Drawing for the job (mm, zero at the part's lowest x, y, z). A direction names the side the tool comes from. Coordinates: 2 decimals unless noted, no trailing zeros. Write each loop counter-clockwise with the first axis right and the second up, starting at its lowest first coordinate (ties: lowest second). Pieces come first, ordered by that corner, then holes. Notation, with made-up numbers: M 43,29.5 L 68,29.5 A27 cw 68,66.5 Z; hole C 81.25,-36 d4. An arc over 180 degrees is marked long. Use a Markdown table: item, result. Add a question column.
Q1. Tool access for the marked faces 5 and 6: list every direction of +Z, -Z, +X, -X, +Y, -Y with a clear straight run to the whole face (end or side of a thin tool).
Q2. Wall check: L1, parallel to X at y = 4, z = 19.05; L2, parallel to Z at x = 38.1, y = 3; L3, parallel to Z at x = 27, y = 13.5. Give the ranges that are in metal, low to high. Write a range as from..to.
Q3. Slice it at B-B on x = 38.1. Write the cut outline in (y, z).
Q4. Mould opens along Z. For the marked faces 1, 2, 3 and 4 say: released by +Z, released by -Z, zero draft, split by the parting line, or undercut.
Q5. Slice it at C-C on y = 17. Write the cut outline in (x, z).
Q6. Slice it at A-A on z = 19.05. Write the cut outline in (x, y), then the cut area to 3 significant figures.
Q7. Pin check, flat tips, straight feed: pin 1 Ø3 at (y, z) = (21.5, 9) entering from +X; pin 2 Ø5 at (x, y) = (28, 27) entering from +Z; pin 3 Ø3 at (x, y) = (28, 13.5) entering from +Z; pin 4 Ø7.5 at (x, z) = (16, 15.5) entering from +Y. Stop position of each tip, or through.
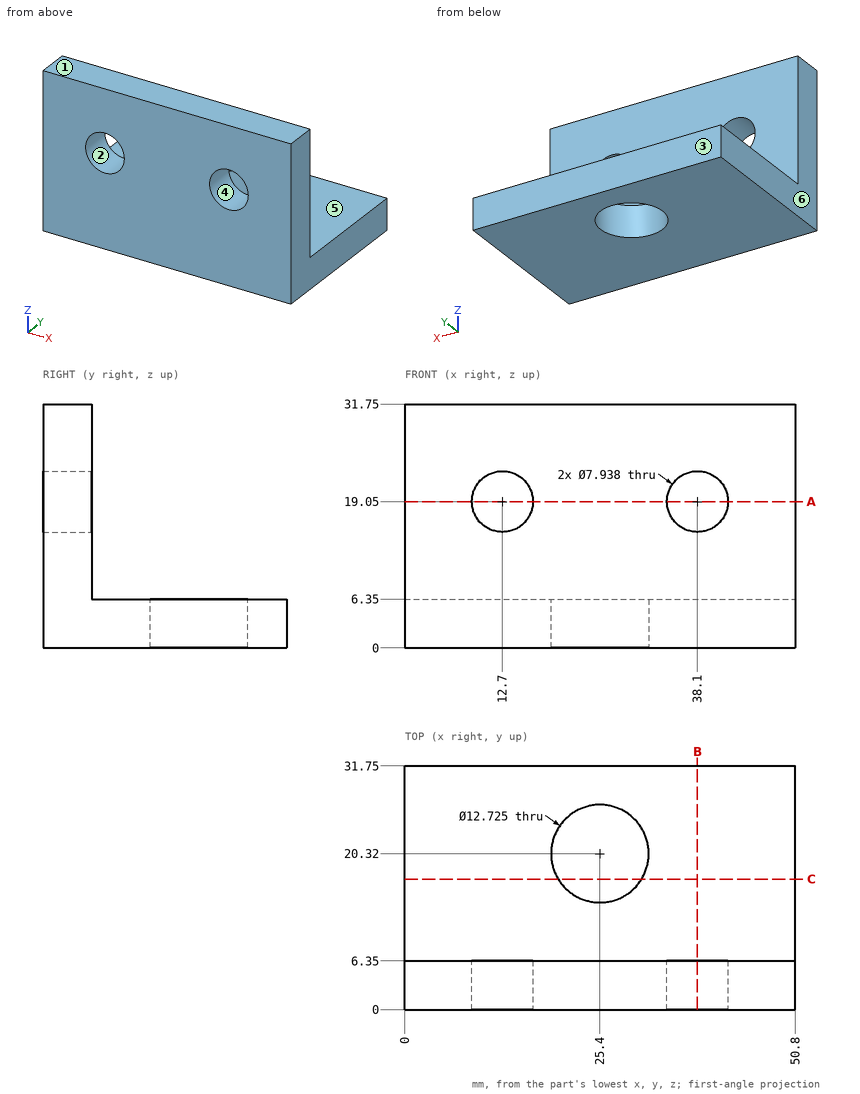
Recorded:
| question | item | result |
|---|---|---|
| 1 | face 5 | +Z, +X, -X, +Y |
| 1 | face 6 | +Z, -Z, -X, +Y, -Y |
| 2 | L1 | 0..8.73, 16.67..34.13, 42.07..50.8 |
| 2 | L2 | 0..15.08, 23.02..31.75 |
| 2 | L3 | 0..6.35 |
| 3 | outline | M 0,0 L 31.75,0 L 31.75,6.35 L 6.35,6.35 L 6.35,15.08 L 0,15.08 Z; M 0,23.02 L 6.35,23.02 L 6.35,31.75 L 0,31.75 Z |
| 4 | face 1 | released by +Z |
| 4 | face 2 | undercut |
| 4 | face 3 | zero draft |
| 4 | face 4 | undercut |
| 5 | outline | M 0,0 L 19.97,0 L 19.97,6.35 L 0,6.35 Z; M 30.83,0 L 50.8,0 L 50.8,6.35 L 30.83,6.35 Z |
| 6 | outline | M 0,0 L 8.73,0 L 8.73,6.35 L 0,6.35 Z; M 16.67,0 L 34.13,0 L 34.13,6.35 L 16.67,6.35 Z; M 42.07,0 L 50.8,0 L 50.8,6.35 L 42.07,6.35 Z |
| 6 | area | 222 mm² |
| 7 | pin 1 | through |
| 7 | pin 2 | z = 6.35 |
| 7 | pin 3 | z = 6.35 |
| 7 | pin 4 | y = 6.35 |
